The model under review builds one solid part; all positions refer to its coordinate system, in mm. Face numbers are marked on the shaded views. A direction names the side the tool comes from. Coordinates: 2 decimals unless noted, no trailing zeros. Order: outer loops, then holes, each group sorted by start corner. A loop starts at its lowest first (then second) coordinate and runs counter-clockwise, first axis right, second up. Notation, with made-up numbers: (-30.5, 67) - (13.5, 67) arc R26 ccw to (13.5, 85) - close; hole circle Ø7 at (89.5, 11). An arc over 180 degrees is marked (long way). Answer in a Markdown table with one row per item.
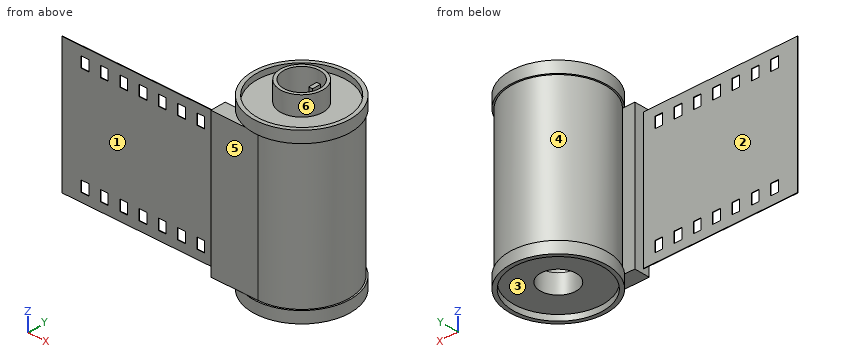
```python
from build123d import *

# Parameters (mm, degrees)
F1_DEPTH  = 18.65
F4_R      = 4.65
F5_DEPTH  = 5
F7_DEPTH  = 7
F10_R     = 5.5
F10_R_2   = 4.7
F11_DEPTH = 5
F12_R     = 4.7
F13_DEPTH = 9.5
F15_DEPTH = 11.5
F17_W     = 40
F17_H     = 35
F17_W_2   = 2
F17_H_2   = 2.75
F18_DEPTH = 0.14


with BuildPart() as f1:
    # F0 (on Top) → F1 (new body, symmetric)
    with BuildSketch(Plane.XY):
        with BuildLine():
            Line((-12.2, -12.2), (0, -12.2))
            ThreePointArc((0, -12.2), (4.9396356141, 11.1552678139), (-9.0332718325, -8.2))
            Line((-9.0332718325, -8.2), (-12.2, -8.2))
            Line((-12.2, -8.2), (-12.2, -12.2))
        make_face()
    extrude(amount=F1_DEPTH, both=True)

    # F2 (on Front) → F3 (revolve)
    with BuildSketch(Plane.XZ):
        Polygon((12.6, -18.65), (0, -18.65), (0, -20.15), (11.6, -20.15), (11.6, -21.65), (12.6, -21.65), align=None)
    revolve(axis=Axis((0, 0, -19.4), (0, 0, -1)))

    # F4 (on face) → F5 (cut)
    with BuildSketch(Plane(origin=(0, 0, -20.15), x_dir=(1, 0, 0), z_dir=(0, 0, -1))):
        Circle(F4_R)
    extrude(amount=-F5_DEPTH, mode=Mode.SUBTRACT)

    # F6 (on face) → F7 (cut)
    with BuildSketch(Plane(origin=(0, 0, -15.15), x_dir=(1, 0, 0), z_dir=(0, 0, -1))):
        with BuildLine():
            Line((-0.5, -4.6230401253), (-0.5, 4.6230401253))
            ThreePointArc((-0.5, 4.6230401253), (-4.65, 0), (-0.5, -4.6230401253))
        make_face()
        with BuildLine():
            ThreePointArc((4.65, 0), (3.4603106797, 3.1062437123), (0.5, 4.6230401253))
            Line((0.5, 4.6230401253), (0.5, -4.6230401253))
            ThreePointArc((0.5, -4.6230401253), (3.4603106797, -3.1062437123), (4.65, 0))
        make_face()
    extrude(amount=-F7_DEPTH, mode=Mode.SUBTRACT)

    # F8 (on Front) → F9 (revolve)
    with BuildSketch(Plane.XZ):
        Polygon((0, 20.15), (0, 18.65), (12.6, 18.65), (12.6, 21.65), (11.6, 21.65), (11.6, 20.15), align=None)
    revolve(axis=Axis((0, 0, 19.4), (0, 0, -1)))

    # F10 (on face) → F11 (join)
    with BuildSketch(Plane.XY.offset(20.15)):
        Circle(F10_R)
        Circle(F10_R_2, mode=Mode.SUBTRACT)
    extrude(amount=F11_DEPTH)

    # F12 (on face) → F13 (cut)
    with BuildSketch(Plane.XY.offset(20.15)):
        Circle(F12_R)
    extrude(amount=-F13_DEPTH, mode=Mode.SUBTRACT)

    # F14 (on face) → F15 (join)
    with BuildSketch(Plane.XY.offset(10.65)):
        with BuildLine():
            ThreePointArc((0.5, 4.6733285782), (0, 4.7), (-0.5, 4.6733285782))
            Line((-0.5, 4.6733285782), (-0.5, 2.5))
            Line((-0.5, 2.5), (0.5, 2.5))
            Line((0.5, 2.5), (0.5, 4.6733285782))
        make_face()
        with BuildLine():
            ThreePointArc((-0.5, -4.6733285782), (0, -4.7), (0.5, -4.6733285782))
            Line((0.5, -4.6733285782), (0.5, -2.5))
            Line((0.5, -2.5), (-0.5, -2.5))
            Line((-0.5, -2.5), (-0.5, -4.6733285782))
        make_face()
    extrude(amount=F15_DEPTH)

    # F17 (on offset) → F18 (join)
    with BuildSketch(Plane.XZ.offset(10.55)):
        with Locations((-32.2, 0)):
            Rectangle(F17_W, F17_H)
        with Locations((-46.2, -13.875)):
            Rectangle(F17_W_2, F17_H_2, mode=Mode.SUBTRACT)
        with Locations((-41.2, -13.875)):
            Rectangle(F17_W_2, F17_H_2, mode=Mode.SUBTRACT)
        with Locations((-36.2, -13.875)):
            Rectangle(F17_W_2, F17_H_2, mode=Mode.SUBTRACT)
        with Locations((-31.2, -13.875)):
            Rectangle(F17_W_2, F17_H_2, mode=Mode.SUBTRACT)
        with Locations((-26.2, -13.875)):
            Rectangle(F17_W_2, F17_H_2, mode=Mode.SUBTRACT)
        with Locations((-21.2, -13.875)):
            Rectangle(F17_W_2, F17_H_2, mode=Mode.SUBTRACT)
        with Locations((-16.2, -13.875)):
            Rectangle(F17_W_2, F17_H_2, mode=Mode.SUBTRACT)
        with Locations((-46.2, 13.875)):
            Rectangle(F17_W_2, F17_H_2, mode=Mode.SUBTRACT)
        with Locations((-41.2, 13.875)):
            Rectangle(F17_W_2, F17_H_2, mode=Mode.SUBTRACT)
        with Locations((-36.2, 13.875)):
            Rectangle(F17_W_2, F17_H_2, mode=Mode.SUBTRACT)
        with Locations((-31.2, 13.875)):
            Rectangle(F17_W_2, F17_H_2, mode=Mode.SUBTRACT)
        with Locations((-26.2, 13.875)):
            Rectangle(F17_W_2, F17_H_2, mode=Mode.SUBTRACT)
        with Locations((-21.2, 13.875)):
            Rectangle(F17_W_2, F17_H_2, mode=Mode.SUBTRACT)
        with Locations((-16.2, 13.875)):
            Rectangle(F17_W_2, F17_H_2, mode=Mode.SUBTRACT)
    extrude(amount=F18_DEPTH)


solid = f1.part
```
Item 1: To check wall thickness, follow line 1 (Y direction, x = 0, z = 21.2); line 2 (Z direction, x = -5.5, y = 11); line 3 (Y direction, x = 0, z = -17.9). State the ranges of each line that lie inside material, in increasing order. Write a range as from..to.
Check values:
| item | result |
|---|---|
| line 1 | -12.6..-11.6, -5.5..-2.5, 2.5..5.5, 11.6..12.6 |
| line 2 | -21.65..-18.65, 18.65..21.65 |
| line 3 | -12.2..-4.65, 4.65..12.2 |
Item 2: We need section C-C, the plane x = -23. Write out the cut boundary in (y, z), then the cut area to 3 significant figures.
Check values:
| item | result |
|---|---|
| outline | (-10.69, -17.5) - (-10.55, -17.5) - (-10.55, 17.5) - (-10.69, 17.5) - close |
| area | 4.90 mm^2 |
Item 3: We need section A-A, the plane z = 4. Write out the cut boundary in (x, y).
Check values:
| item | result |
|---|---|
| outline | (-52.2, -10.69) - (-12.2, -10.69) - (-12.2, -12.2) - (0, -12.2) arc R12.2 ccw (long way) to (-9.03, -8.2) - (-12.2, -8.2) - (-12.2, -10.55) - (-52.2, -10.55) - close |
Item 4: Mouldability with a two-part tool opening along Y and no side actions: class the marked faces 1, 2 and 3 as +Y half, -Y half, draft (parallel to the pull), parting line (faces both ways), or undercut.
Check values:
| item | result |
|---|---|
| face 1 | -Y half |
| face 2 | +Y half |
| face 3 | undercut |
Item 5: Tool access review of the marked faces 4, 5 and 6: name each direction out of +Z, -Z, +X, -X, +Y, -Y from which nothing blocks a thin tool from reaching the whole face with its end or side.
Check values:
| item | result |
|---|---|
| face 4 | none |
| face 5 | +X, -X, -Y |
| face 6 | +Z |
Item 6: Clearance check with flat-ended pins moving along their axes: pin 1 Ø3 at (x, z) = (-12, -10) entering from +Y; pin 2 Ø6 at (x, z) = (-5.5, -2.5) entering from -Y; pin 3 Ø2 at (x, z) = (-37.5, 9.5) entering from -Y. State where each tip first meets the part, or that it passes through.
Check values:
| item | result |
|---|---|
| pin 1 | y = 6.21 |
| pin 2 | y = -12.2 |
| pin 3 | y = -10.69 |
